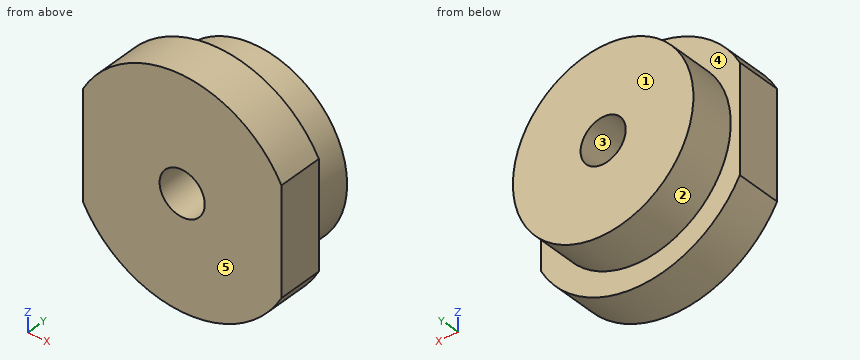
```python
from build123d import *

# Parameters (mm, degrees)
SKIZZE1_R                       = 12.5
AUFSATZ_LINEAR_AUSTRAGEN1_DEPTH = 5
SKIZZE2_R                       = 10
AUFSATZ_LINEAR_AUSTRAGEN2_DEPTH = 5
SKIZZE3_R                       = 2.5
SCHNITT_LINEAR_AUSTRAGEN1_DEPTH = 11


with BuildPart() as part:
    # Skizze1 → Aufsatz-Linear austragen1 (new body)
    with BuildSketch(Plane(origin=(0, 0, 0), x_dir=(1, 0, 0), z_dir=(0, 1, 0))):
        Circle(SKIZZE1_R)
    extrude(amount=AUFSATZ_LINEAR_AUSTRAGEN1_DEPTH)

    # Skizze2 → Aufsatz-Linear austragen2 (add)
    with BuildSketch(Plane(origin=(0, 5, 0), x_dir=(1, 0, 0), z_dir=(0, 1, 0))):
        Circle(SKIZZE2_R)
    extrude(amount=AUFSATZ_LINEAR_AUSTRAGEN2_DEPTH)

    # Skizze3 → Schnitt-Linear austragen1 (cut, through all)
    with BuildSketch(Plane(origin=(0, 10, 0), x_dir=(1, 0, 0), z_dir=(0, 1, 0))):
        Circle(SKIZZE3_R)
        with BuildLine():
            Line((-11, 5.937171044), (-11, -5.937171044))
            ThreePointArc((-11, -5.937171044), (-12.5, 0), (-11, 5.937171044))
        make_face()
        with BuildLine():
            Line((11, 5.937171044), (11, -5.937171044))
            ThreePointArc((11, -5.937171044), (12.5, 0), (11, 5.937171044))
        make_face()
    extrude(amount=-SCHNITT_LINEAR_AUSTRAGEN1_DEPTH, mode=Mode.SUBTRACT)


solid = part.part
```
Geometry check sheet. Reference: the model listing, model coordinates, mm. Face numbers are marked on the shaded views. A direction names the side the tool comes from. Coordinates: 2 decimals unless noted, no trailing zeros. Order: outer loops, then holes, each group sorted by start corner. A loop starts at its lowest first (then second) coordinate and runs counter-clockwise, first axis right, second up. Notation, with made-up numbers: M 26,-32 L 63,-32 A8 cw 63,-24 Z; hole C 81,43 d1. An arc over 180 degrees is marked long. One line per question, with ' | ' between items. Start each with the question number.
Item 1: Cross-section at B-B on z = 0. Enter the section's corners in (x, y), then the cut area to 3 significant figures.
Item 2: Material ranges on L1, parallel to Z at x = 0, y = 7.25; L2, parallel to X at y = 4.25, z = 0, recorded low to high. Write a range as [from, to].
Item 3: Gauge pin test, flat ends, axial feed: pin 1 (2 mm diameter, centred on y = 9, z = -4.5, fed in from -X); pin 2 (6 mm diameter, centred on x = -8, y = 5.5, fed in from +Z); pin 3 (5 mm diameter, centred on x = -8, y = 4, fed in from -Z) (3 decimals). Record the tip position at first contact, or that the pin passes through.
Item 4: Set-up check for the marked faces 4 and 5: record each of +Z, -Z, +X, -X, +Y, -Y from which the full face is reachable in a straight line by a thin tool's end or side.
Item 5: Cross-section at D-D on x = 9.25. Enter the section's corners in (y, z), then the cut area to 3 significant figures.
Item 6: Cross-section at C-C on y = 3.75. Enter the section's corners in (x, z), then the cut area to 3 significant figures.
Item 7: Draft check along X on the marked faces 1, 2 and 3. Enter one of: pulls with the +X half, pulls with the -X half, needs draft (parallel to the pull), parting line crosses it, or undercut.
Item 8: Cross-section at A-A on x = 0. Enter the section's corners in (y, z), then the cut area to 3 significant figures.
Findings:
1) outline: M -11,0 L -2.5,0 L -2.5,10 L -10,10 L -10,5 L -11,5 Z; M 2.5,0 L 11,0 L 11,5 L 10,5 L 10,10 L 2.5,10 Z | area: 160 mm²
2) L1: z = [-10, -2.5], [2.5, 10] | L2: x = [-11, -2.5], [2.5, 11]
3) pin 1: stops at x = -9.37 | pin 2: stops at z = 11.44 | pin 3: stops at z = -11.225
4) face 4: +Y | face 5: +Z, -Z, +X, -X, -Y
5) outline: M 0,-8.41 L 5,-8.41 L 5,-3.8 L 10,-3.8 L 10,3.8 L 5,3.8 L 5,8.41 L 0,8.41 Z | area: 122 mm²
6) outline: M -11,-5.94 A12.5 ccw 11,-5.94 L 11,5.94 A12.5 ccw -11,5.94 Z; hole C 0,0 d5 | area: 447 mm²
7) face 1: needs draft | face 2: parting line crosses it | face 3: undercut
8) outline: M 0,-12.5 L 5,-12.5 L 5,-10 L 10,-10 L 10,-2.5 L 0,-2.5 Z; M 0,2.5 L 10,2.5 L 10,10 L 5,10 L 5,12.5 L 0,12.5 Z | area: 175 mm²
